Part model, mm, in its own coordinate system. A direction names the side the tool comes from. Round coordinates to 2 decimals unless told otherwise and drop trailing zeros. Loops run counter-clockwise (first coordinate to the right, second up) from the corner with the lowest first, then second, coordinate; pieces in that order, holes last.
1) Band-saw the part on A-A, the plane x = -63.5. Write the cut outline in (y, z), then the cut area to 3 significant figures.
2) Band-saw the part on D-D, the plane y = 28. Write the cut outline in (x, z).
3) Drop flat-ended pins along their axis: P1, Ø6, axis at x = -11.5, y = 54.5, coming from the -Z side; P2, Ø6, axis at x = 0, z = 63.5, coming from the -Y side; P3, Ø3, axis at x = 37.5, y = 23, coming from the -Z side; P4, Ø2, axis at x = 22.5, y = 21.5, coming from the +Z side. Give the stop position or say it passes through.
4) Probe line 1 (Y direction, x = -18, z = 21.5); line 2 (Z direction, x = 63.5, y = 3.5); line 3 (Y direction, x = -40, z = 44). List the from-to ranges inside material, lowest first.
5) Band-saw the part on C-C, the plane x = -25.5. Write the cut outline in (y, z), then the cut area to 3 significant figures.
6) 3-axis set-ups, long thin cutter, end or side, ignore diameter. For faces 1 (the cylindrical face through (49.592, 59.746, 11.012)), 2 (the cylindrical face through (49.592, 112.311, 11.012)), 3 (the cylindrical face through (-52.85, 3.13, -30.1)): which of +Z, -Z, +X, -X, +Y, -Y reach the whole face in a straight line?
7) Mould opens along X. For faces 4 (the flat face through (20, 120.65, 47)), 5 (the cylindrical face through (57.695, 3.131, -31.869)), 6 (the cylindrical face through (42.503, 3.219, 55.431)), 7 (the cylindrical face through (33.9, 117.43, -53.35)) say: +X half, -X half, draft (parallel to the pull), parting line (faces both ways), or undercut.
from build123d import *

# Parameters (mm, degrees)
SKETCH4_W                  = 30.48
SKETCH4_H                  = 2.54
F_3_0_213_DIAMETER_HOLE2_D = 5.4102


with BuildPart() as part:
    # Sketch1 → Chamber (revolve)
    with BuildSketch(Plane(origin=(0, 0, 0), x_dir=(0, 0, -1), z_dir=(1, 0, 0))):
        Polygon((57.15, 6.35), (57.15, 114.3), (69.85, 114.3), (69.85, 120.65), (57.15, 120.65), (50.8, 120.65), (50.8, 114.3), (50.8, 6.35), (50.8, 0), (57.15, 0), (69.85, 0), (69.85, 6.35), align=None)
    revolve(axis=Axis((0, 0, 0), (0, 1, 0)))

    # Sketch4 → Turbulence Rings (revolve)
    with BuildSketch(Plane(origin=(0, 0, 0), x_dir=(0, 0, -1), z_dir=(1, 0, 0))):
        with Locations((35.56, 102.931657822)):
            Rectangle(SKETCH4_W, SKETCH4_H)
        with Locations((35.56, 17.718342178)):
            Rectangle(SKETCH4_W, SKETCH4_H)
    revolve(axis=Axis((0, 0, 0), (0, 1, 0)))

    # #3 (0.213) Diameter Hole2 (through all)
    with Locations(Plane(origin=(0, 120.65, 0), x_dir=(1, 0, 0), z_dir=(0, 1, 0))):
        with Locations((0, 0), (-63.5, 0), (-54.99261314, 31.75), (-31.75, 54.99261314), (0, 63.5), (31.75, 54.99261314), (54.99261314, 31.75), (63.5, 0), (54.99261314, -31.75), (31.75, -54.99261314), (0, -63.5), (-31.75, -54.99261314), (-54.99261314, -31.75)):
            Hole(F_3_0_213_DIAMETER_HOLE2_D / 2)


solid = part.part
Reported:
1. outline: (0, -29.1) - (6.35, -29.1) - (6.35, -2.71) - (0, -2.71) - close; (0, 2.71) - (6.35, 2.71) - (6.35, 29.1) - (0, 29.1) - close; (114.3, -29.1) - (120.65, -29.1) - (120.65, -2.71) - (114.3, -2.71) - close; (114.3, 2.71) - (120.65, 2.71) - (120.65, 29.1) - (114.3, 29.1) - close
1. area: 670 mm2
2. outline: circle Ø114.3 at (0, 0); hole circle Ø101.6 at (0, 0)
3. P1: stops at z = -56.51
3. P2: stops at y = 0
3. P3: stops at z = -44.39
3. P4: stops at z = 52.95
4. line 1: y = 16.45 to 18.99, 101.66 to 104.2
4. line 2: z = -29.1 to -2.71, 2.71 to 29.1
4. line 3: y = 0 to 6.35, 114.3 to 120.65
5. outline: (0, -65.03) - (6.35, -65.03) - (6.35, -51.15) - (114.3, -51.15) - (114.3, -65.03) - (120.65, -65.03) - (120.65, -43.94) - (104.2, -43.94) - (104.2, 43.94) - (120.65, 43.94) - (120.65, 65.03) - (114.3, 65.03) - (114.3, 51.15) - (6.35, 51.15) - (6.35, 65.03) - (0, 65.03) - (0, 43.94) - (16.45, 43.94) - (16.45, -43.94) - (0, -43.94) - close; hole (18.99, -43.94) - (101.66, -43.94) - (101.66, 43.94) - (18.99, 43.94) - close
5. area: 2,540 mm2
6. face 1: none
6. face 2: +Y
6. face 3: +Y, -Y
7. face 4: draft
7. face 5: undercut
7. face 6: parting line
7. face 7: undercut
